Geometry check sheet. Reference: the model listing, model coordinates, mm. A direction names the side the tool comes from. Coordinates: 2 decimals unless noted, no trailing zeros. Loops run counter-clockwise (first coordinate to the right, second up) from the corner with the lowest first, then second, coordinate; pieces in that order, holes last. Notation, with made-up numbers: (37.5, -23.75) - (88.5, -23.75) arc R29 ccw to (88.5, -2.75) - close; hole circle Ø7 at (86.5, 49.5). An arc over 180 degrees is marked (long way). Write item = value, one per line. Start each with the question number.
from build123d import *

# Parameters (mm, degrees)
SKETCH1_R                = 15
SKETCH1_R_2              = 2.55
BOSS_EXTRUDE1_DEPTH      = 20
BOSS_EXTRUDE2_DEPTH      = 15
BOSS_EXTRUDE2_DEPTH_BACK = 15


with BuildPart() as part:
    # Sketch1 → Boss-Extrude1 (new body)
    with BuildSketch(Plane.XY):
        Circle(SKETCH1_R)
        Circle(SKETCH1_R_2, mode=Mode.SUBTRACT)
    extrude(amount=BOSS_EXTRUDE1_DEPTH)

    # Sketch2 → Boss-Extrude2 (add, two sides)
    with BuildSketch(Plane(origin=(0, 0, 0), x_dir=(1, 0, 0), z_dir=(0, 1, 0))) as boss_extrude2_sk:
        with BuildLine():
            Line((50, -35.949524979), (50, -30))
            ThreePointArc((50, -30), (0, -19.050475021), (-50, -30))
            Line((-50, -30), (-50, -35.949524979))
            ThreePointArc((-50, -35.949524979), (0, -25), (50, -35.949524979))
        make_face()
    extrude(amount=BOSS_EXTRUDE2_DEPTH)
    extrude(boss_extrude2_sk.sketch, amount=-BOSS_EXTRUDE2_DEPTH_BACK)


solid = part.part
(1) Scan lines: line 1 (X direction, y = 0, z = 6); line 2 (Z direction, x = 1, y = 6.5). Record each from-to range of solid material in increasing order.
(2) Depth check by flat-ended pin: pin 1 (2 mm diameter, centred on y = 8, z = 18, fed in from -X); pin 2 (10 mm diameter, centred on x = 18, y = -6, fed in from +Z); pin 3 (1 mm diameter, centred on y = -10.5, z = 18.5, fed in from -X). Enter the tip coordinate at first touch or a pass-through.
(3) Sectioned sample at C-C on x = 33.5. Enter the section's corners in (y, z), plus the area to 3 significant figures.
(4) Sectioned sample at B-B on z = 15.5. Enter the section's corners in (x, y).
(5) Sectioned sample at D-D on y = 7. Enter the section's corners in (x, z), plus the area to 3 significant figures.
(6) Sectioned sample at A-A on y = 0. Enter the section's corners in (x, z).
(7) Tool access check on faces 4 (the face through (0.04, 0.02, 19.05)), 5 (the face through (-50, 0, 33)). Record the directions out of +Z, -Z, +X, -X, +Y, -Y that give a thin tool (end or side, any length) a straight path to the whole face; none if there is none.
(8) Draft check along Y on faces 1 (the face through (-1, 15, 24)), 2 (the face through (3, 0, 0)), 3 (the face through (1.18, -2.26, 9.41)). Enter one of: pulls with the +Y half, pulls with the -Y half, needs draft (parallel to the pull), parting line crosses it, or undercut.
Working result:
q1.line_1 = -15 to -2.55, 2.55 to 15
q1.line_2 = 0 to 25
q2.pin_1 = -13.27
q2.pin_2 = 27.23
q2.pin_3 = -11.18
q3.outline = (-15, 23.84) - (15, 23.84) - (15, 29.79) - (-15, 29.79) - close
q3.area = 178 mm2
q4.outline = circle Ø30 at (0, 0); hole circle Ø5.1 at (0, 0)
q5.outline = (-50, 30) arc R119.63 ccw to (-13.27, 19.79) - (-13.27, 0) - (13.27, 0) - (13.27, 19.79) arc R119.63 ccw to (50, 30) - (50, 35.95) arc R119.63 cw to (-50, 35.95) - close
q5.area = 1,110 mm2
q6.outline = (-50, 30) arc R119.63 ccw to (-15, 19.99) - (-15, 0) - (-2.55, 0) - (-2.55, 19.08) arc R119.63 ccw to (2.55, 19.08) - (2.55, 0) - (15, 0) - (15, 19.99) arc R119.63 ccw to (50, 30) - (50, 35.95) arc R119.63 cw to (-50, 35.95) - close
q7.face_4 = -Z
q7.face_5 = +Z, -Z, -X, +Y, -Y
q8.face_1 = pulls with the +Y half
q8.face_2 = needs draft
q8.face_3 = undercut
